from build123d import *

# Parameters (mm, degrees)
F0_W     = 127
F0_H     = 50.8
F0_R     = 12.6365
F0_R_2   = 9.525
F0_R_3   = 8.9535
F1_DEPTH = 25.4


with BuildPart() as f1:
    # F0 (on Front) → F1 (new body)
    with BuildSketch(Plane.XZ):
        with Locations((-58.905346, 25.4)):
            Rectangle(F0_W, F0_H)
        with Locations((-95.625527, 30.434817)):
            Circle(F0_R, mode=Mode.SUBTRACT)
        with Locations((-64.432904, 32.12858)):
            Circle(F0_R_2, mode=Mode.SUBTRACT)
        with Locations((-35.189819, 32.12858)):
            Circle(F0_R_3, mode=Mode.SUBTRACT)
        with BuildLine():
            ThreePointArc((4.594654, 0), (182.394654, 25.4), (4.594654, 50.8))
            Line((4.594654, 50.8), (4.594654, 0))
        make_face()
    extrude(amount=F1_DEPTH)


solid = f1.part
Here's how the part is built. I have some questions about the finished solid (model axes, mm). A direction names the side the tool comes from. Round coordinates to 2 decimals unless told otherwise and drop trailing zeros. Order: outer loops, then holes, each group sorted by start corner. A loop starts at its lowest first (then second) coordinate and runs counter-clockwise, first axis right, second up. Notation, with made-up numbers: M -16.75,1 L 3.25,1 A17 cw 3.25,19 Z; hole C 28.25,42.25 d10. An arc over 180 degrees is marked long. Return JSON: item names as keys, results as strings. Group by question number.
1. If we section it at D-D on x = -6: List the corners of the cut face in (y, z) for me, then the cut area to 3 significant figures.
2. If we section it at A-A on y = -12: State how many separate pieces and enclosed holes the cut face has, then the cut area to 3 significant figures.
3. Please list where these lines run through material, in increasing order: probe 1 along Z at (x, y) = (-95, -23.5); probe 2 along X at (y, z) = (-12.25, 29); probe 3 along Z at (x, y) = (-13, -24.5).
4. If we mould it in two halves opening along X, with no side actions, what happens to faces 4 (the face through (-73.95, -12.52, 32.55)), 5 (the face through (182.32, -12.52, 21.77)), 6 (the face through (62, -25.4, 27))? For each: pulls with the +X half, pulls with the -X half, needs draft (parallel to the pull), parting line crosses it, or undercut.
5. On a 3-axis mill with a long thin cutter (end or side, diameter ignored), from which of +Z, -Z, +X, -X, +Y, -Y can I reach the whole of each face in a straight line? I mean faces 1 (the face through (-60, -13, 0)), 2 (the face through (-122.405, -13, 25)), 3 (the face through (-60, -13, 50.8)). Say none if no direction works.
6. I'm going to push flat-ended pins straight in: pin 1 Ø8 at (y, z) = (-20.5, 27) entering from +X; pin 2 Ø10 at (x, y) = (137, -21.5) entering from +Z; pin 3 Ø7.5 at (x, y) = (-39, -10.5) entering from -Z. Where does each tip first touch, or does it pass through?
7. If we section it at C-C on z = 96.5: List the corners of the cut face in (x, y) for me.
8. If we section it at B-B on x = -92.5: List the corners of the cut face in (y, z) for me, then the cut area to 3 significant figures.
Reply:
{
 "1": {"outline": "M -25.4,0 L 0,0 L 0,50.8 L -25.4,50.8 Z", "area": "1,290 mm^2"},
 "2": {"separate pieces": "1", "enclosed holes": "3", "area": "31,100 mm^2"},
 "3": {"probe 1": "0 to 17.81, 43.06 to 50.8", "probe 2": "-122.41 to -108.18, -83.07 to -73.43, -55.44 to -43.58, -26.8 to 182.32", "probe 3": "0 to 50.8"},
 "4": {"face 4": "undercut", "face 5": "parting line crosses it", "face 6": "needs draft"},
 "5": {"face 1": "-Z, -X, +Y, -Y", "face 2": "+Z, -Z, -X, +Y, -Y", "face 3": "+Z, -X, +Y, -Y"},
 "6": {"pin 1": "x = 182.39", "pin 2": "z = 106.66", "pin 3": "z = 0"},
 "7": {"outline": "M 35.34,-25.4 L 148.02,-25.4 L 148.02,0 L 35.34,0 Z"},
 "8": {"outline": "M -25.4,0 L 0,0 L 0,18.19 L -25.4,18.19 Z; M -25.4,42.68 L 0,42.68 L 0,50.8 L -25.4,50.8 Z", "area": "668 mm^2"}
}
